from build123d import *

# Parameters (mm, degrees)
F0_W          = 61.4048474937
F0_H          = 2
F1_DEPTH      = 30
F4_DEPTH      = 31
F4_DEPTH_BACK = 30.4048474937
F5_DEPTH      = 25


with BuildPart() as f1:
    # F0 (on Front) → F1 (new body)
    with BuildSketch(Plane.XZ):
        with BuildLine():
            Line((-37.0734768147, 14.5654241689), (-39.1259005615, 9.7618792294))
            ThreePointArc((-39.1259005615, 9.7618792294), (-39.0833815375, 9.2899496059), (-38.6661121219, 9.0654241689))
            Line((-38.6661121219, 9.0654241689), (-17.9661121219, 9.0654241689))
            Line((-17.9661121219, 9.0654241689), (-17.9661121219, 10.7654241689))
            Line((-17.9661121219, 10.7654241689), (1.1191584926, 10.7654241689))
            Line((1.1191584926, 10.7654241689), (1.1191584926, 9.0654241689))
            Line((1.1191584926, 9.0654241689), (21.8191584926, 9.0654241689))
            ThreePointArc((21.8191584926, 9.0654241689), (22.2364279081, 9.2899496059), (22.2789469322, 9.7618792294))
            Line((22.2789469322, 9.7618792294), (20.2265231853, 14.5654241689))
            Line((20.2265231853, 14.5654241689), (22.2789469322, 19.6776874363))
            Line((22.2789469322, 19.6776874363), (-39.1259005615, 19.6776874363))
            Line((-39.1259005615, 19.6776874363), (-37.0734768147, 14.5654241689))
        make_face()
        with Locations((-8.4234768147, 20.6776874363)):
            Rectangle(F0_W, F0_H)
    extrude(amount=F1_DEPTH)

    # F3 (on offset) → F4 (join, two sides)
    with BuildSketch(Plane.YZ.offset(-8.7210530678)) as f4_sk:
        with BuildLine():
            Line((138.8979104789, 38.204113167), (89.6575228283, 29.5217042836))
            Line((89.6575228283, 29.5217042836), (0, 21.6776874363))
            Line((0, 21.6776874363), (0, 19.6776874363))
            Line((0, 19.6776874363), (90.0055822498, 27.5522234792))
            Line((90.0055822498, 27.5522234792), (139.2452068342, 36.234497661))
            ThreePointArc((139.2452068342, 36.234497661), (140.0563664095, 37.3929535916), (138.8979104789, 38.204113167))
        make_face()
    extrude(amount=F4_DEPTH)
    extrude(f4_sk.sketch, amount=-F4_DEPTH_BACK)

    # F3 (on offset) → F5 (join, symmetric)
    with BuildSketch(Plane.YZ.offset(-8.7210530678)):
        with BuildLine():
            Line((138.8979104789, 38.204113167), (89.6575228283, 29.5217042836))
            Line((89.6575228283, 29.5217042836), (0, 21.6776874363))
            Line((0, 21.6776874363), (0, 19.6776874363))
            Line((0, 19.6776874363), (90.0055822498, 27.5522234792))
            Line((90.0055822498, 27.5522234792), (139.2452068342, 36.234497661))
            ThreePointArc((139.2452068342, 36.234497661), (140.0563664095, 37.3929535916), (138.8979104789, 38.204113167))
        make_face()
        Polygon((90.0055822498, 27.5522234792), (0, 19.6776874363), (0, 15.6776874363), align=None)
    extrude(amount=F5_DEPTH, both=True)


solid = f1.part
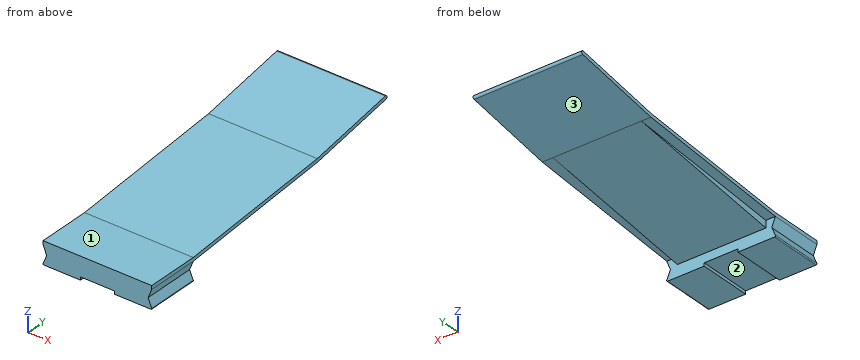
Part model, mm, in its own coordinate system. Face numbers are marked on the shaded views. A direction names the side the tool comes from. Round coordinates to 2 decimals unless told otherwise and drop trailing zeros. Write each loop counter-clockwise with the first axis right and the second up, starting at its lowest first coordinate (ties: lowest second). Pieces come first, ordered by that corner, then holes. Notation, with made-up numbers: (43.25, 28.25) - (62.25, 28.25) arc R9 cw to (62.25, 43.25) - close; hole circle Ø10 at (-0.5, 17.5). An arc over 180 degrees is marked (long way). Use CSV: the item, a comma, the result in double quotes.
Item 1: Flat gauge pins, fed straight in: P1, Ø9.5, axis at y = 65.5, z = 29.5, coming from the +X side; P2, Ø8, axis at x = -25.5, y = 1, coming from the +Z side; P3, Ø9, axis at x = -14.5, y = -17, coming from the +Z side. Where does each tip first touch, or does it go through?
Results list:
P1,"stops at x = 22.28"
P2,"stops at z = 22.12"
P3,"stops at z = 21.68"
Item 2: Slice it at B-B, the plane y = 72.5. Write the cut outline in (x, z), then the cut area to 3 significant figures.
Results list:
outline,"(-39.13, 26.02) - (-33.72, 26.02) - (-33.72, 25.24) - (16.28, 25.24) - (16.28, 26.02) - (22.28, 26.02) - (22.28, 28.02) - (-39.13, 28.02) - close"
area,"162 mm²"
Item 3: Tool access for the marked faces 1, 2 and 3: list every direction of +Z, -Z, +X, -X, +Y, -Y with a clear straight run to the whole face (end or side of a thin tool).
Results list:
face 1,"+Z, +X, -X, -Y"
face 2,"-Z, +Y, -Y"
face 3,"-Z, +X, -X, +Y"
Item 4: Slice it at D-D, the plane x = 4. Write the cut outline in (y, z), then the cut area to 3 significant figures.
Results list:
outline,"(-30, 9.07) - (0, 9.07) - (0, 15.68) - (90.01, 27.55) - (139.25, 36.23) arc R1 ccw to (138.9, 38.2) - (89.66, 29.52) - (0, 21.68) - (-30, 21.68) - close"
area,"840 mm²"
Item 5: Wall check: L1, parallel to Y at x = -36, z = 11; L2, parallel to X at y = 29, z = 20; L3, parallel to Z at x = -17.5, y = -11. Give the ranges that are in metal, low to high.
Results list:
L1,"y = -30 to 0"
L2,"x = -33.72 to 16.28"
L3,"z = 10.77 to 21.68"
Item 6: Slice it at A-A, the plane x = -2.5. Write the cut outline in (y, z).
Results list:
outline,"(-30, 10.77) - (0, 10.77) - (0, 15.68) - (90.01, 27.55) - (139.25, 36.23) arc R1 ccw to (138.9, 38.2) - (89.66, 29.52) - (0, 21.68) - (-30, 21.68) - close"
Item 7: Slice it at C-C, the plane z = 18. Write the cut outline in (x, y), then the cut area to 3 significant figures.
Results list:
outline,"(-38.45, -30) - (21.61, -30) - (21.61, 0) - (16.28, 0) - (16.28, 17.6) - (-33.72, 17.6) - (-33.72, 0) - (-38.45, 0) - close"
area,"2,680 mm²"
